Source: CAD feature listing. Evaluate the final solid. Frame: model axes, mm. A direction names the side the tool comes from. Give positions to 0.01 mm unless a question says otherwise; leave off trailing zeros. Write each loop counter-clockwise with the first axis right and the second up, starting at its lowest first coordinate (ties: lowest second). Pieces come first, ordered by that corner, then holes. Notation, with made-up numbers: (75, 57) -> (110, 57) arc R6 ccw to (110, 68) -> close; hole circle Ø5 at (18, -16.75). An arc over 180 degrees is marked (long way). Answer as a JSON object with one key per item and string values. Group by question number.
Item 1: Ray query, probe 1 along Z at (x, y) = (-74.25, 15); probe 2 along X at (y, z) = (56, 0.5); probe 3 along X at (y, z) = (75, 2). Return the intervals inside material, ascending. Write a range as from..to.
Item 2: Access query for faces 4 (the face through (-78, 39, 1)), 5 (the face through (-76, 39, -4)), 6 (the face through (-71, 0, 0)). Directions: +Z, -Z, +X, -X, +Y, -Y. A direction counts if a zero-diameter tool reaches every point of the face in a straight line with its end or side. Return the directions, or none.
Item 3: Section query B-B on y = 33.5. Return the cut outline in (x, z), plus the area to 3 significant figures.
Item 4: Section query D-D on x = -72.25. Return the cut outline in (y, z).
Item 5: Pull-direction query (Z, two-part tool) for faces 1 (the face through (-73.223, 39, 0)), 2 (the face through (-76, 39, 4)), 3 (the face through (-83.223, 39, 3)); classes: pulls with the +Z half, pulls with the -Z half, needs draft (parallel to the pull), parting line crosses it, or undercut.
Item 6: First-contact query: pin 1 Ø3 at (y, z) = (42.5, -0.5) entering from +X; pin 2 Ø0.6 at (y, z) = (55, 0) entering from -X; pin 3 Ø8 at (x, y) = (-70.5, 62.5) entering from -Z. Flat tips, straight axial feed; report the tip coordinate or a pass-through.
Item 7: Section query C-C on z = -3.25. Return the cut outline in (x, y) (3 decimals), plus the area to 3 significant figures.
Item 8: Section query A-A on x = -75.5. Return the cut outline in (y, z).
from build123d import *

# Parameters (mm, degrees)
BOSS_EXTRUDE1_DEPTH      = 80
M1_2X0_25_TAPPED_HOLE2_D = 0.95


with BuildPart() as part:
    # Sketch1 → Boss-Extrude1 (new body)
    with BuildSketch(Plane(origin=(0, 0, 0), x_dir=(1, 0, 0), z_dir=(0, 1, 0))):
        with BuildLine():
            Line((-64.012503946, -11.287131548), (-67.140480461, -11.838678203))
            ThreePointArc((-67.140480461, -11.838678203), (-67.722822081, -7.932947987), (-68.07746332, -4))
            Line((-68.07746332, -4), (-68.222773013, -4))
            Line((-68.222773013, -4), (-83.222773013, -4))
            Line((-83.222773013, -4), (-83.222773013, -1))
            Line((-83.222773013, -1), (-73.222773013, -1))
            Line((-73.222773013, -1), (-73.222773013, 1))
            Line((-73.222773013, 1), (-83.222773013, 1))
            Line((-83.222773013, 1), (-83.222773013, 4))
            Line((-83.222773013, 4), (-68.222773013, 4))
            Line((-68.222773013, 4), (-68.093710355, 4))
            ThreePointArc((-68.093710355, 4), (-67.754779073, 7.936674143), (-67.187770434, 11.847016701))
            Line((-67.187770434, 11.847016701), (-64.012503946, 11.287131548))
            ThreePointArc((-64.012503946, 11.287131548), (-65, 0), (-64.012503946, -11.287131548))
        make_face()
    extrude(amount=BOSS_EXTRUDE1_DEPTH)

    # M1.2x0.25 Tapped Hole2 (through all)
    with Locations(Plane.XY.offset(4)):
        with Locations((-78.222773013, 75), (-78.222773013, 40), (-78.222773013, 5)):
            Hole(M1_2X0_25_TAPPED_HOLE2_D / 2)


solid = part.part
Worked answers:
{
 "1": {"probe 1": "-4..-1, 1..4", "probe 2": "-73.22..-65", "probe 3": "-83.22..-78.7, -77.75..-64.97"},
 "2": {"face 4": "-X, +Y, -Y", "face 5": "-Z, -X, +Y, -Y", "face 6": "+Z, -Z, +X, -X, -Y"},
 "3": {"outline": "(-83.22, -4) -> (-68.09, -4) arc R68 ccw to (-67.19, -11.85) -> (-64.01, -11.29) arc R65 cw to (-64.01, 11.29) -> (-67.14, 11.84) arc R68 ccw to (-68.08, 4) -> (-83.22, 4) -> (-83.22, 1) -> (-73.22, 1) -> (-73.22, -1) -> (-83.22, -1) -> close", "area": "175 mm^2"},
 "4": {"outline": "(0, -4) -> (80, -4) -> (80, 4) -> (0, 4) -> close"},
 "5": {"face 1": "undercut", "face 2": "pulls with the +Z half", "face 3": "needs draft"},
 "6": {"pin 1": "x = -64.97", "pin 2": "x = -73.22", "pin 3": "z = -11.85"},
 "7": {"outline": "(-83.223, 0) -> (-64.919, 0) -> (-64.919, 80) -> (-83.223, 80) -> close; hole circle Ø0.95 at (-78.223, 5); hole circle Ø0.95 at (-78.223, 40); hole circle Ø0.95 at (-78.223, 75)", "area": "1,460 mm^2"},
 "8": {"outline": "(0, -4) -> (80, -4) -> (80, -1) -> (0, -1) -> close; (0, 1) -> (80, 1) -> (80, 4) -> (0, 4) -> close"}
}
